Source: three-view drawing plus pictorial views. Frame: mm from the lowest corner of the part. A direction names the side the tool comes from. Give positions to 0.01 mm unless a question says otherwise; leave off trailing zeros. Write each loop counter-clockwise with the first axis right and the second up, starting at its lowest first coordinate (ties: lowest second). Pieces come first, ordered by that corner, then holes. Notation, with made-up numbers: M 68,-8.5 L 88,-8.5 A7 ccw 88,2.5 Z; hole C 68.5,52 d9. An arc over 180 degrees is marked long. One line per question, with ' | ' between items.
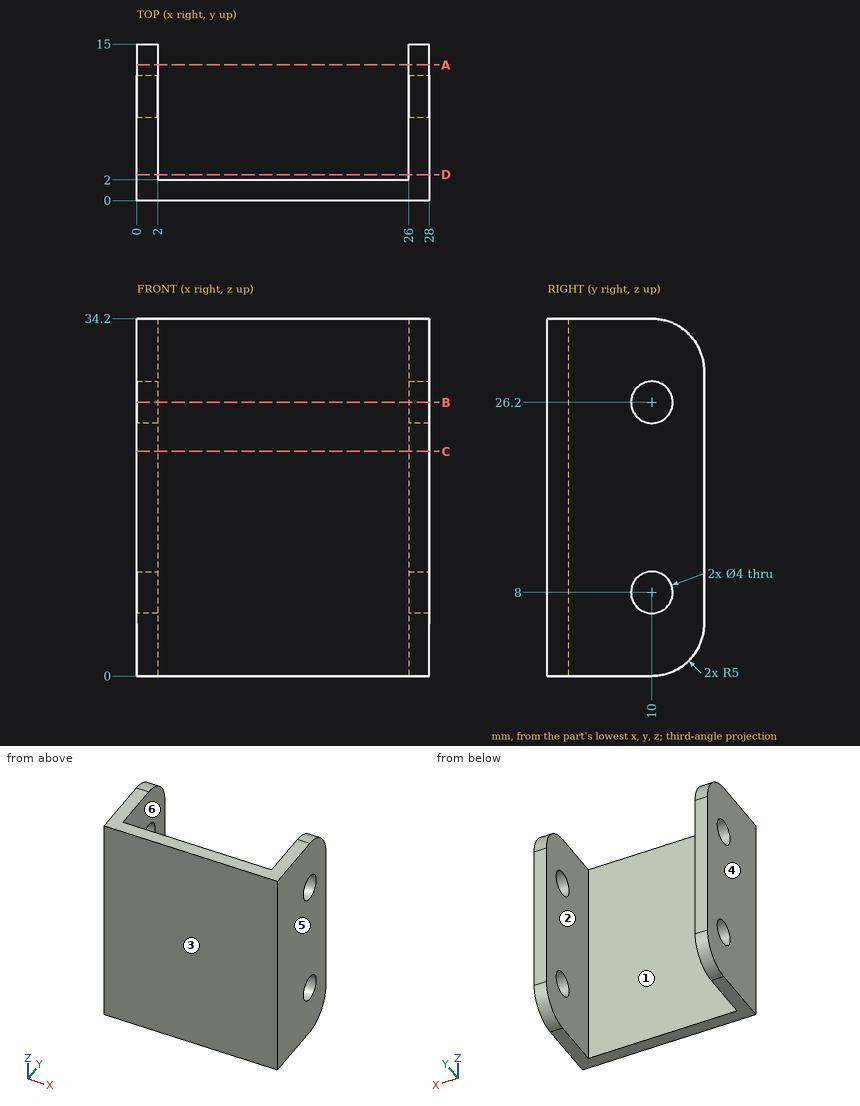
(1) Material intervals for L1, parallel to X at y = 2.25, z = 28; L2, parallel to Y at x = 26.85, z = 26.2; L3, parallel to Y at x = 7.5, z = 2, sorted ascending. Write a range as [from, to].
Working result:
L1: x = [0, 2], [26, 28] | L2: y = [0, 8], [12, 15] | L3: y = [0, 2]
(2) Cut plane D-D, the plane y = 2.5. Return loops of the section in (x, z), then the cut area to 3 significant figures.
Working result:
outline: M 0,0 L 2,0 L 2,34.2 L 0,34.2 Z; M 26,0 L 28,0 L 28,34.2 L 26,34.2 Z | area: 137 mm^2
(3) Cut plane A-A, the plane y = 13. Return loops of the section in (x, z).
Working result:
outline: M 0,1 L 2,1 L 2,33.2 L 0,33.2 Z; M 26,1 L 28,1 L 28,33.2 L 26,33.2 Z
(4) Set-up query: the marked faces 5 and 6. Return all of +Z, -Z, +X, -X, +Y, -Y with unobstructed straight access to the full face (end or side cutting, diameter ignored); none if empty.
Working result:
face 5: +Z, -Z, +X, +Y, -Y | face 6: +Z, -Z, +Y
(5) Draft query along X for the marked faces 1, 2, 3 and 4. Return one class per face: released by +X, released by -X, zero draft, split by the parting line, or undercut.
Working result:
face 1: undercut | face 2: undercut | face 3: zero draft | face 4: released by -X
(6) Cut plane B-B, the plane z = 26.2. Return loops of the section in (x, y).
Working result:
outline: M 0,0 L 28,0 L 28,8 L 26,8 L 26,2 L 2,2 L 2,8 L 0,8 Z; M 0,12 L 2,12 L 2,15 L 0,15 Z; M 26,12 L 28,12 L 28,15 L 26,15 Z
(7) First-contact query: P1, Ø2.5, axis at y = 10, z = 26.2, coming from the -X side; P2, Ø4, axis at x = 11, y = 3, coming from the +Z side; P3, Ø6, axis at x = 11.5, z = 12.5, coming from the +Y side. Flat tips, straight axial feed; report the tip coordinate or a pass-through.
Working result:
P1: passes through | P2: stops at z = 34.2 | P3: stops at y = 2
(8) Cut plane C-C, the plane z = 21.5. Return loops of the section in (x, y), then the cut area to 3 significant figures.
Working result:
outline: M 0,0 L 28,0 L 28,15 L 26,15 L 26,2 L 2,2 L 2,15 L 0,15 Z | area: 108 mm^2
